```python
from build123d import *

# Parameters (mm, degrees)
SKETCH1_R                                        = 139.7
BOSS_EXTRUDE1_DEPTH                              = 6.35
SKETCH2_R                                        = 134.112
BOSS_EXTRUDE2_DEPTH                              = 3
BOSS_EXTRUDE3_DEPTH                              = 5
SKETCH37_R                                       = 177.8
CUT_EXTRUDE1_DEPTH                               = 268.317994245
CBORE_FOR_M4_HEX_HEAD_MACHINE_SCREW3_D           = 4.3
CBORE_FOR_M4_HEX_HEAD_MACHINE_SCREW3_CBORE_D     = 10.59
CBORE_FOR_M4_HEX_HEAD_MACHINE_SCREW3_CBORE_DEPTH = 3
CIRPATTERN1_COUNT                                = 4
F_5_8_0_625_DIAMETER_HOLE1_D                     = 15.875
SKETCH73_R                                       = 139.7
SKETCH73_R_2                                     = 134.112
BOSS_EXTRUDE4_DEPTH                              = 3
SKETCH74_R                                       = 3.81
SKETCH74_R_2                                     = 2.5
CUT_EXTRUDE5_DEPTH                               = 198.786760174
SKETCH75_R                                       = 21.59
CUT_EXTRUDE6_DEPTH                               = 1.8
SKETCH76_R                                       = 10.795
CUT_EXTRUDE7_DEPTH                               = 198.786760174
CBORE_FOR_M5_HEX_HEAD_MACHINE_SCREW1_D           = 5.3
CBORE_FOR_M5_HEX_HEAD_MACHINE_SCREW1_CBORE_D     = 11.71
CBORE_FOR_M5_HEX_HEAD_MACHINE_SCREW1_CBORE_DEPTH = 3.8
CBORE_FOR_M5_HEX_HEAD_BOLT1_D                    = 5.3
CBORE_FOR_M5_HEX_HEAD_BOLT1_CBORE_D              = 12.24
CBORE_FOR_M5_HEX_HEAD_BOLT1_CBORE_DEPTH          = 3.58
SKETCH84_R                                       = 5.855
BOSS_EXTRUDE6_DEPTH                              = 9.35
SKETCH85_R                                       = 5.295
SKETCH85_R_2                                     = 2.15
SKETCH85_R_3                                     = 21.59
SKETCH85_R_4                                     = 10.795
BOSS_EXTRUDE7_DEPTH                              = 3


with BuildPart() as part:
    # Sketch1 → Boss-Extrude1 (new body)
    with BuildSketch(Plane(origin=(0, 0, 0), x_dir=(1, 0, 0), z_dir=(0, 1, 0))):
        with Locations(Location((0, 0, 0), (0, 0, 270))):
            Circle(SKETCH1_R)
    extrude(amount=BOSS_EXTRUDE1_DEPTH)

    # Sketch2 → Boss-Extrude2 (add)
    with BuildSketch(Plane.XZ):
        with Locations(Location((0, 0, 0), (0, 0, 270))):
            Circle(SKETCH2_R)
    extrude(amount=BOSS_EXTRUDE2_DEPTH)

    # Sketch3 → Boss-Extrude3 (add, symmetric)
    with BuildSketch(Plane.XY):
        with BuildLine():
            Line((-38.1, 95.25), (-38.1, 6.35))
            Line((-38.1, 6.35), (-139.7, 6.35))
            Line((-139.7, 6.35), (-164.11656703, 72.845121962))
            ThreePointArc((-164.11656703, 72.845121962), (-114.47811829, 159.246393895), (-38.1, 95.25))
        make_face()
    extrude(amount=BOSS_EXTRUDE3_DEPTH, both=True)

    # Sketch37 → Cut-Extrude1 (cut, through all)
    with BuildSketch(Plane(origin=(0, 6.35, 0), x_dir=(1, 0, 0), z_dir=(0, 1, 0))):
        Circle(SKETCH37_R)
    extrude(amount=CUT_EXTRUDE1_DEPTH, mode=Mode.SUBTRACT)

    # CBORE for M4 Hex Head Machine Screw3 (through all)
    with Locations(Plane(origin=(0, 6.35, 0), x_dir=(1, 0, 0), z_dir=(0, 1, 0))):
        with Locations((52.109857404, 67.910888344)):
            cbore_for_m4_hex_head_machine_screw3 = CounterBoreHole(CBORE_FOR_M4_HEX_HEAD_MACHINE_SCREW3_D / 2, CBORE_FOR_M4_HEX_HEAD_MACHINE_SCREW3_CBORE_D / 2, CBORE_FOR_M4_HEX_HEAD_MACHINE_SCREW3_CBORE_DEPTH)

    # CirPattern1: CBORE for M4 Hex Head Machine Screw3 ×4 about axis
    cirpattern1_axis = Axis((0, 0, 0), (0, 1, 0))
    for i in range(1, CIRPATTERN1_COUNT):
        add(cbore_for_m4_hex_head_machine_screw3.rotate(cirpattern1_axis, i * 360 / CIRPATTERN1_COUNT), mode=Mode.SUBTRACT)

    # 5/8 (0.625) Diameter Hole1 (through all)
    with Locations(Plane(origin=(0, 6.35, 0), x_dir=(1, 0, 0), z_dir=(0, 1, 0))):
        with Locations((-99.914329603, 0)):
            Hole(F_5_8_0_625_DIAMETER_HOLE1_D / 2)

    # Sketch73 → Boss-Extrude4 (add)
    with BuildSketch(Plane.XZ):
        with Locations(Location((0, 0, 0), (0, 0, 270))):
            Circle(SKETCH73_R)
        Circle(SKETCH73_R_2, mode=Mode.SUBTRACT)
    extrude(amount=BOSS_EXTRUDE4_DEPTH)

    # Sketch74 → Cut-Extrude5 (cut, through all)
    with BuildSketch(Plane(origin=(0, 6.35, 0), x_dir=(1, 0, 0), z_dir=(0, 1, 0))):
        with Locations(Location((10.959973331, -22.913729172, 0), (0, 0, 270))):
            Circle(SKETCH74_R)
        with Locations(Location((34.529973331, -46.483729172, 0), (0, 0, 270))):
            Circle(SKETCH74_R_2)
        with Locations(Location((-12.610026669, -46.483729172, 0), (0, 0, 270))):
            Circle(SKETCH74_R_2)
        with Locations(Location((-12.610026669, 0.656270828, 0), (0, 0, 270))):
            Circle(SKETCH74_R_2)
        with Locations(Location((34.529973331, 0.656270828, 0), (0, 0, 270))):
            Circle(SKETCH74_R_2)
    extrude(amount=-CUT_EXTRUDE5_DEPTH, mode=Mode.SUBTRACT)

    # Sketch75 → Cut-Extrude6 (cut)
    with BuildSketch(Plane(origin=(0, 6.35, 0), x_dir=(1, 0, 0), z_dir=(0, 1, 0))):
        with Locations(Location((10.959973331, -22.913729172, 0), (0, 0, 270))):
            Circle(SKETCH75_R)
    extrude(amount=-CUT_EXTRUDE6_DEPTH, mode=Mode.SUBTRACT)

    # Sketch76 → Cut-Extrude7 (cut, through all)
    with BuildSketch(Plane.XZ.offset(3)):
        with Locations(Location((10.959973331, 22.913729172, 0), (0, 0, 270))):
            Circle(SKETCH76_R)
    extrude(amount=-CUT_EXTRUDE7_DEPTH, mode=Mode.SUBTRACT)

    # CBORE for M5 Hex Head Machine Screw1 (through all)
    with Locations(Plane(origin=(0, -3, 0), x_dir=(-1, 0, 0), z_dir=(0, -1, 0))):
        with Locations((-35.56, 96.52), (-35.56, 66.04), (-35.56, 35.56), (22.86, 35.56), (22.86, 66.04), (22.86, 96.52)):
            CounterBoreHole(CBORE_FOR_M5_HEX_HEAD_MACHINE_SCREW1_D / 2, CBORE_FOR_M5_HEX_HEAD_MACHINE_SCREW1_CBORE_D / 2, CBORE_FOR_M5_HEX_HEAD_MACHINE_SCREW1_CBORE_DEPTH)

    # CBORE for M5 Hex Head Bolt1 (through all)
    with Locations(Plane(origin=(-79.322298318, -3, -83.174678927), x_dir=(0, 0, -1), z_dir=(0, -1, 0))):
        with Locations((0, 0), (-37.220558849, -13.421994622), (1.981025557, 20.485311492)):
            CounterBoreHole(CBORE_FOR_M5_HEX_HEAD_BOLT1_D / 2, CBORE_FOR_M5_HEX_HEAD_BOLT1_CBORE_D / 2, CBORE_FOR_M5_HEX_HEAD_BOLT1_CBORE_DEPTH)

    # Sketch84 → Boss-Extrude6 (add)
    with BuildSketch(Plane.XZ.offset(3)):
        with Locations((35.56, -66.04)):
            Circle(SKETCH84_R)
        with Locations((-22.86, -66.04)):
            Circle(SKETCH84_R)
    extrude(amount=-BOSS_EXTRUDE6_DEPTH)

    # Sketch85 → Boss-Extrude7 (add)
    # profile 1 of 5: a face of its own
    with BuildSketch(Plane(origin=(0, 6.35, 0), x_dir=(1, 0, 0), z_dir=(0, 1, 0))):
        with Locations((-52.109857404, -67.910888344)):
            Circle(SKETCH85_R)
        with Locations(Location((-52.109857404, -67.910888344, 0), (0, 0, 270))):
            Circle(SKETCH85_R_2, mode=Mode.SUBTRACT)
    # profile 2 of 5: a face of its own
    with BuildSketch(Plane(origin=(0, 6.35, 0), x_dir=(1, 0, 0), z_dir=(0, 1, 0))):
        with Locations((67.910888344, -52.109857404)):
            Circle(SKETCH85_R)
        with Locations(Location((67.910888344, -52.109857404, 0), (0, 0, 270))):
            Circle(SKETCH85_R_2, mode=Mode.SUBTRACT)
    # profile 3 of 5: a face of its own
    with BuildSketch(Plane(origin=(0, 6.35, 0), x_dir=(1, 0, 0), z_dir=(0, 1, 0))):
        with Locations((10.959973331, -22.913729172)):
            Circle(SKETCH85_R_3)
        with Locations(Location((10.959973331, -22.913729172, 0), (0, 0, 90))):
            Circle(SKETCH85_R_4, mode=Mode.SUBTRACT)
    # profile 4 of 5: a face of its own
    with BuildSketch(Plane(origin=(0, 6.35, 0), x_dir=(1, 0, 0), z_dir=(0, 1, 0))):
        with Locations((52.109857404, 67.910888344)):
            Circle(SKETCH85_R)
        with Locations(Location((52.109857404, 67.910888344, 0), (0, 0, 270))):
            Circle(SKETCH85_R_2, mode=Mode.SUBTRACT)
    # profile 5 of 5: a face of its own
    with BuildSketch(Plane(origin=(0, 6.35, 0), x_dir=(1, 0, 0), z_dir=(0, 1, 0))):
        with Locations((-67.910888344, 52.109857404)):
            Circle(SKETCH85_R)
        with Locations(Location((-67.910888344, 52.109857404, 0), (0, 0, 270))):
            Circle(SKETCH85_R_2, mode=Mode.SUBTRACT)
    extrude(amount=-BOSS_EXTRUDE7_DEPTH)


solid = part.part
```
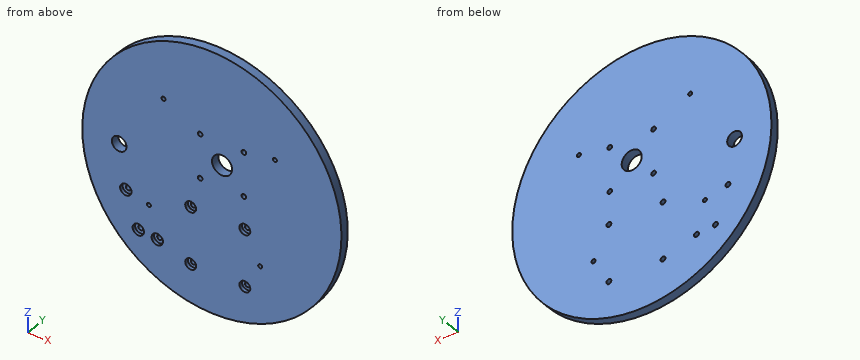
CAD build for the part. Positions are in the model's coordinates, mm. Round coordinates to 2 decimals unless told otherwise and drop trailing zeros. Loops run counter-clockwise (first coordinate to the right, second up) from the corner with the lowest first, then second, coordinate; pieces in that order, holes last. Notation, with made-up numbers: M 32.5,31 L 40.5,31 A23 ccw 40.5,55 Z; hole C 7.25,30 d6. An arc over 180 degrees is marked long. Use a Markdown table: item, result. Add a question column.
(1) Cut at A-A (x = 84.5). Give the cut face in (y, z).
(2) Flat gauge pins, fed straight in: pin 1 (4 mm diameter, centred on x = -92.74, z = -45.95, fed in from -Y); pin 2 (1.5 mm diameter, centred on x = -61.5, y = 2, fed in from +Z); pin 3 (4 mm diameter, centred on x = -87.5, y = -1, fed in from +Z); pin 4 (11 mm diameter, centred on x = -79.32, z = -83.17, fed in from -Y). Where does each tip first touch, or does it go through?
(3) Drill centre lines: line 1 (X direction, y = -1.7, z = -35.56) (3 decimals); line 2 (Z direction, x = -22.86, y = -1.45) (3 decimals); line 3 (Z direction, x = 35.56, y = 2.3). Where is each one in solid material? Low to high.
(4) Cut at B-B (z = 78). Give the cut face in (x, y), and give its area (3 significant figures).
Geometry says:
| question | item | result |
|---|---|---|
| 1 | outline | M -3,-111.25 L 6.35,-111.25 L 6.35,111.25 L -3,111.25 Z |
| 2 | pin 1 | passes through |
| 2 | pin 2 | stops at z = 125.8 |
| 2 | pin 3 | stops at z = 110.48 |
| 2 | pin 4 | stops at y = 0.58 |
| 3 | line 1 | x = -135.098 to -28.715, -17.005 to 29.705, 41.415 to 135.098 |
| 3 | line 2 | z = -137.817 to -102.375, -90.665 to -41.415, -29.705 to 137.817 |
| 3 | line 3 | z = -135.1 to -99.17, -93.87 to -38.21, -32.91 to -2.93, 1.62 to 44.21, 48.76 to 135.1 |
| 4 | outline | M -115.9,-3 L 115.9,-3 L 115.9,6.35 L -115.9,6.35 Z |
| 4 | area | 2,170 mm² |
